```python
from build123d import *

# Parameters (mm, degrees)
SKETCH_R        = 11.3
SKETCH_R_2      = 1.6
SKETCH_R_3      = 3.2
PAD_DEPTH       = 15
SKETCH001_R     = 3.2
POCKET_DEPTH    = 4
SKETCH002_R     = 5.4
POCKET001_DEPTH = 4
FILLET_R        = 4
CHAMFER_SIZE    = 0.4
CHAMFER001_SIZE = 0.2
CHAMFER002_SIZE = 0.2
CHAMFER003_SIZE = 0.4


with BuildPart() as part:
    # Sketch → Pad (new body)
    with BuildSketch(Plane.XY):
        Polygon((20, 30), (20, 50.15), (62.3, 50.15), (62.3, 30), (82.3, 30), (82.3, 0), (0, 0), (0, 30), align=None)
        with Locations((41.15, 29)):
            Circle(SKETCH_R, mode=Mode.SUBTRACT)
        with Locations((25.65, 44.5)):
            Circle(SKETCH_R_2, mode=Mode.SUBTRACT)
        with Locations((25.65, 13.5)):
            Circle(SKETCH_R_2, mode=Mode.SUBTRACT)
        with Locations((56.65, 44.5)):
            Circle(SKETCH_R_2, mode=Mode.SUBTRACT)
        with Locations((56.65, 13.5)):
            Circle(SKETCH_R_2, mode=Mode.SUBTRACT)
        with Locations((11.15, 10)):
            Circle(SKETCH_R_3, mode=Mode.SUBTRACT)
        with Locations((67.35, 10)):
            Circle(SKETCH_R_3, mode=Mode.SUBTRACT)
        with Locations((78.75, 10)):
            Circle(SKETCH_R_3, mode=Mode.SUBTRACT)
    extrude(amount=PAD_DEPTH)

    # Sketch001 (on Face18 of Pad) → Pocket (cut)
    with BuildSketch(Plane.XY.offset(15)):
        with Locations((25.65, 44.5)):
            Circle(SKETCH001_R)
        with Locations((56.65, 44.5)):
            Circle(SKETCH001_R)
        with Locations((56.65, 13.5)):
            Circle(SKETCH001_R)
        with Locations((25.65, 13.5)):
            Circle(SKETCH001_R)
    extrude(amount=-POCKET_DEPTH, mode=Mode.SUBTRACT)

    # Sketch002 (on Face4 of Pocket) → Pocket001 (cut)
    with BuildSketch(Plane(origin=(0, 0, 0), x_dir=(1, 0, 0), z_dir=(0, 0, -1))):
        with Locations((11.15, -10)):
            Circle(SKETCH002_R)
        with Locations((67.35, -10)):
            Circle(SKETCH002_R)
        with Locations((78.75, -10)):
            Circle(SKETCH002_R)
    extrude(amount=-POCKET001_DEPTH, mode=Mode.SUBTRACT)

    # Fillet
    fillet_edges = [part.edges().sort_by_distance(p)[0] for p in [
        (0, 30, 7.5),
        (0, 0, 7.5),
        (82.3, 0, 7.5),
        (82.3, 30, 7.5),
        (62.3, 30, 7.5),
        (62.3, 50.15, 7.5),
        (20, 50.15, 7.5),
        (20, 30, 7.5),
    ]]
    fillet(fillet_edges, radius=FILLET_R)

    # Chamfer
    chamfer_edges = [part.edges().sort_by_distance(p)[0] for p in [
        (64.15, 10, 15),
        (53.45, 44.5, 15),
        (29.85, 29, 15),
        (22.45, 44.5, 15),
        (22.45, 13.5, 15),
        (7.95, 10, 15),
    ]]
    chamfer(chamfer_edges, length=CHAMFER_SIZE)

    # Chamfer001
    chamfer001_edges = [part.edges().sort_by_distance(p)[0] for p in [
        (81.128427, 1.171573, 15),
        (41.15, 0, 15),
        (1.171573, 1.171573, 15),
        (0, 15, 15),
        (1.171573, 28.828427, 15),
        (10, 30, 15),
        (18.828427, 31.171573, 15),
        (20, 40.075, 15),
        (21.171573, 48.978427, 15),
        (41.15, 50.15, 15),
        (61.128427, 48.978427, 15),
        (62.3, 40.075, 15),
        (63.471573, 31.171573, 15),
        (72.3, 30, 15),
        (81.128427, 28.828427, 15),
    ]]
    chamfer(chamfer001_edges, length=CHAMFER001_SIZE)

    # Chamfer002
    chamfer002_edges = [part.edges().sort_by_distance(p)[0] for p in [
        (10, 30, 0),
        (1.171573, 28.828427, 0),
        (18.828427, 31.171573, 0),
        (0, 15, 0),
        (20, 40.075, 0),
        (1.171573, 1.171573, 0),
        (21.171573, 48.978427, 0),
        (41.15, 0, 0),
        (41.15, 50.15, 0),
        (81.128427, 1.171573, 0),
        (61.128427, 48.978427, 0),
        (82.3, 4.965455, 0),
        (62.3, 40.075, 0),
        (73.35, 10, 0),
        (63.471573, 31.171573, 0),
        (82.3, 20.034545, 0),
        (72.3, 30, 0),
        (81.128427, 28.828427, 0),
        (61.95, 10, 0),
        (55.05, 13.5, 0),
        (24.05, 13.5, 0),
        (5.75, 10, 0),
        (55.05, 44.5, 0),
        (29.85, 29, 0),
        (24.05, 44.5, 0),
    ]]
    chamfer(chamfer002_edges, length=CHAMFER002_SIZE)

    # Chamfer003
    chamfer003_edges = [part.edges().sort_by_distance(p)[0] for p in [
        (82.3, 5.930909, 2.1),
        (82.3, 14.069091, 2.1),
    ]]
    chamfer(chamfer003_edges, length=CHAMFER003_SIZE)


solid = part.part
```
Geometry: final body of the model. Coordinates: model frame, mm. A direction names the side the tool comes from. Coordinates: 2 decimals unless noted, no trailing zeros. Order: outer loops, then holes, each group sorted by start corner. A loop starts at its lowest first (then second) coordinate and runs counter-clockwise, first axis right, second up. Notation, with made-up numbers: (81, -13) - (103, -13) arc R20 ccw to (103, 25) - close; hole circle Ø9 at (-1.5, 10). An arc over 180 degrees is marked (long way). Return JSON: item names as keys, results as strings. Group by question number.
1. Pin query (flat end, axial travel): pin 1 (8.5 mm diameter, centred on x = 78.75, y = 10, fed in from -Z); pin 2 (2 mm diameter, centred on x = 18, y = 40.5, fed in from -Z); pin 3 (4 mm diameter, centred on x = 25.65, y = 44.5, fed in from +Z); pin 4 (6 mm diameter, centred on x = 11, z = 11, fed in from +Y). Return the tip coordinate at first contact, or that it passes through.
2. Pull-direction query (X, two-part tool) for faces 1 (the face through (1.203, 28.859, 7.602)), 2 (the face through (42, 0, 7)), 3 (the face through (26.39, 43.08, 5.52)); classes: pulls with the +X half, pulls with the -X half, needs draft (parallel to the pull), parting line crosses it, or undercut.
3. Cut plane B-B (x = 67.35). Output: boundary loops of the cut face in (y, z).
4. Set-up query: faces 4 (the face through (62.3, 40, 7)), 5 (the face through (28.702, 45.461, 12.825)), 6 (the face through (21.141, 48.947, 7.602)), 7 (the face through (61.955, 9.763, 2.073)). Return all of +Z, -Z, +X, -X, +Y, -Y with unobstructed straight access to the full face (end or side cutting, diameter ignored); none if empty.
5. Cut plane C-C (x = 56.65). Count the separate pieces of the cut face and the enclosed holes in it, plus the area to 3 significant figures.
6. Cut plane A-A (z = 1.25). Output: boundary loops of the cut face in (x, y).
7. Material intervals for line 1 along X through (y, z) = (10, 8.5); line 2 along Y through (x, z) = (56.65, 13.7); line 3 along Y through (x, z) = (57.5, 8.5), sorted ascending. Write a range as [from, to].
Resolved:
{
 "1": {"pin 1": "stops at z = 4", "pin 2": "passes through", "pin 3": "stops at z = 11", "pin 4": "stops at y = 30"},
 "2": {"face 1": "pulls with the -X half", "face 2": "needs draft", "face 3": "undercut"},
 "3": {"outline": "(0, 0.2) - (0.2, 0) - (4.4, 0) - (4.6, 0.2) - (4.6, 4) - (6.8, 4) - (6.8, 14.6) - (6.4, 15) - (0.2, 15) - (0, 14.8) - close; (13.2, 4) - (15.4, 4) - (15.4, 0.2) - (15.6, 0) - (29.8, 0) - (30, 0.2) - (30, 14.8) - (29.8, 15) - (13.6, 15) - (13.2, 14.6) - close"},
 "4": {"face 4": "+Z, -Z, +X, +Y", "face 5": "+Z", "face 6": "+Z, -Z, -X, +Y", "face 7": "-Z"},
 "5": {"separate pieces": "3", "enclosed holes": "0", "area": "630 mm²"},
 "6": {"outline": "(0, 4) arc R4 ccw to (4, 0) - (78.3, 0) arc R4 ccw to (82.3, 4) - (82.3, 5.53) - (81.99, 5.68) arc R5.4 cw (long way) to (81.99, 14.32) - (82.3, 14.47) - (82.3, 26) arc R4 ccw to (78.3, 30) - (66.3, 30) arc R4 cw to (62.3, 34) - (62.3, 46.15) arc R4 ccw to (58.3, 50.15) - (24, 50.15) arc R4 ccw to (20, 46.15) - (20, 34) arc R4 cw to (16, 30) - (4, 30) arc R4 ccw to (0, 26) - close; hole circle Ø10.8 at (11.15, 10); hole circle Ø3.2 at (25.65, 13.5); hole circle Ø3.2 at (25.65, 44.5); hole circle Ø22.6 at (41.15, 29); hole circle Ø3.2 at (56.65, 13.5); hole circle Ø3.2 at (56.65, 44.5); hole circle Ø10.8 at (67.35, 10)"},
 "7": {"line 1": "x = [0, 7.95], [14.35, 64.15], [70.55, 75.55], [81.95, 82.3]", "line 2": "y = [0, 10.3], [16.7, 41.3], [47.7, 50.15]", "line 3": "y = [0, 12.14], [14.86, 43.14], [45.86, 50.15]"}
}
